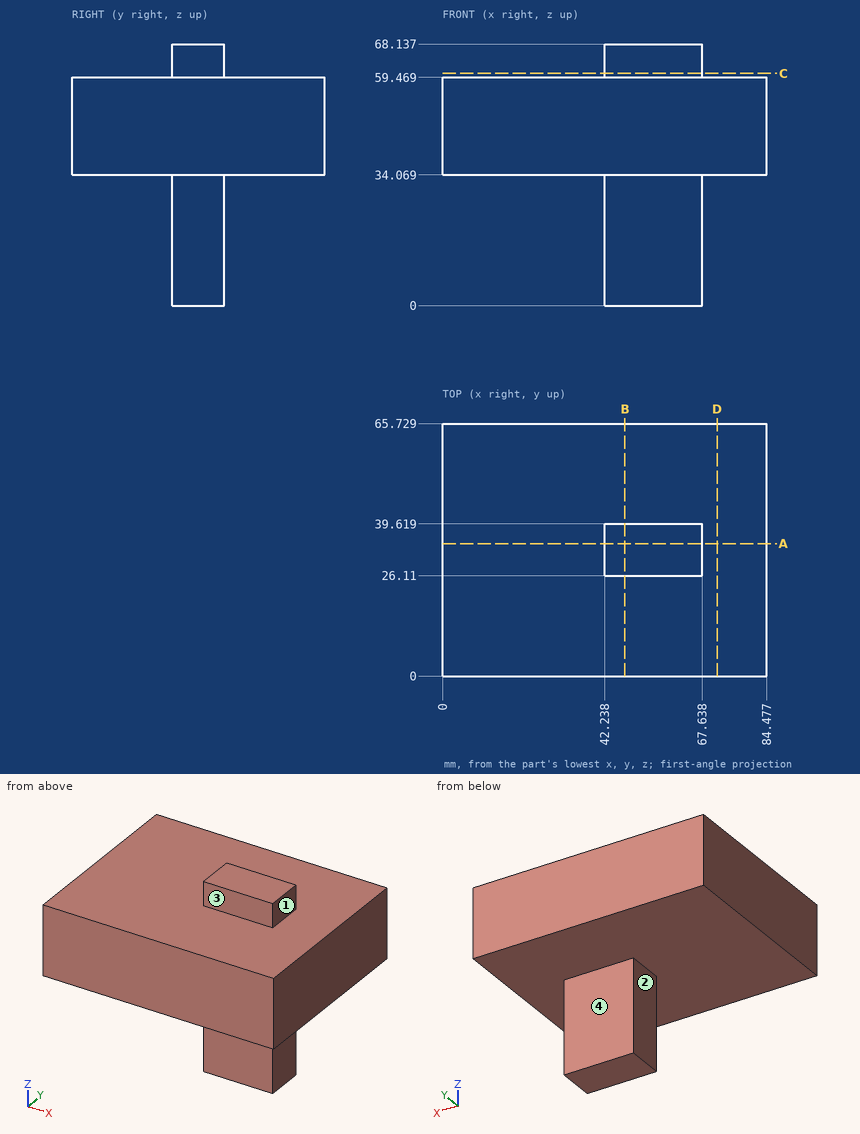
Source: three-view drawing plus pictorial views. Frame: mm from the lowest corner of the part. A direction names the side the tool comes from. Coordinates: 2 decimals unless noted, no trailing zeros. Loops run counter-clockwise (first coordinate to the right, second up) from the corner with the lowest first, then second, coordinate; pieces in that order, holes last. Notation, with made-up numbers: (38.25, 42.25) -> (74.25, 42.25) arc R37 ccw to (74.25, 78.25) -> close; hole circle Ø8 at (11.5, -2). An arc over 180 degrees is marked (long way). Answer in a Markdown table with one row per item. Add a question column.
Q1. Section B-B on x = 47.5. Return the cut outline in (y, z).
Q2. Contact query for flat-ended pins moving along their axis: pin 1 Ø2.5 at (y, z) = (35.5, 62) entering from +X; pin 2 Ø4.5 at (x, z) = (58.5, 64) entering from -Y; pin 3 Ø15 at (y, z) = (34.5, 10.5) entering from -X; pin 4 Ø2 at (x, z) = (35, 61) entering from +Y. Output: stop coordinate, or through.
Q3. Section C-C on z = 60.5. Return the cut outline in (x, y), and give its area (3 significant figures).
Q4. Section D-D on x = 71.5. Return the cut outline in (y, z), and give its area (3 significant figures).
Q5. Reachability of the marked faces 1, 2, 3 and 4 from +Z, -Z, +X, -X, +Y, -Y: full face, straight path, thin tool, end or side. Return the list, or none.
Q6. Section A-A on y = 34.5. Return the cut outline in (x, z), and give its area (3 significant figures).
Q7. Ray query, line 1 along Z through (x, y) = (36, 6.5). Return the intervals inside material, ascending.
Computed values:
| question | item | result |
|---|---|---|
| 1 | outline | (0, 34.07) -> (26.11, 34.07) -> (26.11, 0) -> (39.62, 0) -> (39.62, 34.07) -> (65.73, 34.07) -> (65.73, 59.47) -> (39.62, 59.47) -> (39.62, 68.14) -> (26.11, 68.14) -> (26.11, 59.47) -> (0, 59.47) -> close |
| 2 | pin 1 | stops at x = 67.64 |
| 2 | pin 2 | stops at y = 26.11 |
| 2 | pin 3 | stops at x = 42.24 |
| 2 | pin 4 | passes through |
| 3 | outline | (42.24, 26.11) -> (67.64, 26.11) -> (67.64, 39.62) -> (42.24, 39.62) -> close |
| 3 | area | 343 mm^2 |
| 4 | outline | (0, 34.07) -> (65.73, 34.07) -> (65.73, 59.47) -> (0, 59.47) -> close |
| 4 | area | 1,670 mm^2 |
| 5 | face 1 | +Z, +X, +Y, -Y |
| 5 | face 2 | -Z, -X, +Y, -Y |
| 5 | face 3 | +Z, +X, -X, -Y |
| 5 | face 4 | -Z, +X, -X, +Y |
| 6 | outline | (0, 34.07) -> (42.24, 34.07) -> (42.24, 0) -> (67.64, 0) -> (67.64, 34.07) -> (84.48, 34.07) -> (84.48, 59.47) -> (67.64, 59.47) -> (67.64, 68.14) -> (42.24, 68.14) -> (42.24, 59.47) -> (0, 59.47) -> close |
| 6 | area | 3,230 mm^2 |
| 7 | line 1 | z = 34.07 to 59.47 |
